from build123d import *

# Parameters (mm, degrees)
SKETCH1_W           = 4.75
SKETCH1_H           = 10
SKETCH1_W_2         = 195.25
SKETCH1_H_2         = 75
SKETCH1_W_3         = 10
SKETCH1_H_3         = 6
SKETCH1_H_4         = 35
BOSS_EXTRUDE1_DEPTH = 4.75
SKETCH3_W           = 4.75
SKETCH3_H           = 35
CUT_EXTRUDE2_DEPTH  = 4.75
SKETCH4_W           = 3
SKETCH4_H           = 16
SKETCH4_W_2         = 5.5
SKETCH4_H_2         = 3
CUT_EXTRUDE3_DEPTH  = 4.75
SKETCH5_W           = 10
SKETCH5_H           = 4.75
CUT_EXTRUDE4_DEPTH  = 214.652901923
SKETCH6_R           = 1.5
CUT_EXTRUDE5_DEPTH  = 214.652901923
SKETCH7_W           = 10
SKETCH7_H           = 4.75
BOSS_EXTRUDE2_DEPTH = 4.75
SKETCH8_R           = 2.5
CUT_EXTRUDE6_DEPTH  = 216.366257803
SKETCH9_W           = 3
SKETCH9_H           = 16
SKETCH9_W_2         = 5.5
SKETCH9_H_2         = 3
CUT_EXTRUDE7_DEPTH  = 10


with BuildPart() as part:
    # Sketch1 → Boss-Extrude1 (new body)
    with BuildSketch(Plane(origin=(0, 0, 0), x_dir=(1, 0, 0), z_dir=(0, 1, 0))):
        with Locations((-197.625, 60)):
            Rectangle(SKETCH1_W, SKETCH1_H)
        with Locations((-97.625, 37.5)):
            Rectangle(SKETCH1_W_2, SKETCH1_H_2)
        with Locations((-140.25, -3)):
            Rectangle(SKETCH1_W_3, SKETCH1_H_3)
        with Locations((-97.625, -3)):
            Rectangle(SKETCH1_W_3, SKETCH1_H_3)
        with Locations((-55, -3)):
            Rectangle(SKETCH1_W_3, SKETCH1_H_3)
        with Locations((2.375, 17.5)):
            Rectangle(SKETCH1_W, SKETCH1_H_4)
        with Locations((2.375, 50)):
            Rectangle(SKETCH1_W, SKETCH1_H)
        with Locations((2.375, 70)):
            Rectangle(SKETCH1_W, SKETCH1_H)
        with Locations((-197.625, 40)):
            Rectangle(SKETCH1_W, SKETCH1_H)
    extrude(amount=BOSS_EXTRUDE1_DEPTH)

    # Sketch3 → Cut-Extrude2 (cut)
    with BuildSketch(Plane(origin=(0, 4.75, 0), x_dir=(1, 0, 0), z_dir=(0, 1, 0))):
        with BuildLine():
            Line((-180.25, 35), (-195.25, 35))
            Line((-195.25, 35), (-195.25, 0))
            Line((-195.25, 0), (-150.25, 0))
            Line((-150.25, 0), (-150.25, 5))
            ThreePointArc((-150.25, 5), (-159.036796564, 26.213203436), (-180.25, 35))
        make_face()
        with BuildLine():
            Line((-45, 0), (0, 0))
            Line((0, 0), (0, 35))
            Line((0, 35), (-15, 35))
            ThreePointArc((-15, 35), (-36.213203436, 26.213203436), (-45, 5))
            Line((-45, 5), (-45, 0))
        make_face()
        with Locations((2.375, 17.5)):
            Rectangle(SKETCH3_W, SKETCH3_H)
    extrude(amount=-CUT_EXTRUDE2_DEPTH, mode=Mode.SUBTRACT)

    # Sketch4 → Cut-Extrude3 (cut)
    with BuildSketch(Plane(origin=(0, 4.75, 0), x_dir=(1, 0, 0), z_dir=(0, 1, 0))):
        with Locations((-118.9375, 8)):
            Rectangle(SKETCH4_W, SKETCH4_H)
        with Locations((-76.3125, 8)):
            Rectangle(SKETCH4_W, SKETCH4_H)
        with Locations((-118.9375, 7.5)):
            Rectangle(SKETCH4_W_2, SKETCH4_H_2)
        with Locations((-76.3125, 7.5)):
            Rectangle(SKETCH4_W_2, SKETCH4_H_2)
    extrude(amount=-CUT_EXTRUDE3_DEPTH, mode=Mode.SUBTRACT)

    # Sketch5 → Cut-Extrude4 (cut, through all)
    with BuildSketch(Plane.XZ):
        with Locations((-155.25, -37.375)):
            Rectangle(SKETCH5_W, SKETCH5_H)
        with Locations((-97.625, -37.375)):
            Rectangle(SKETCH5_W, SKETCH5_H)
        with Locations((-40, -37.375)):
            Rectangle(SKETCH5_W, SKETCH5_H)
    extrude(amount=-CUT_EXTRUDE4_DEPTH, mode=Mode.SUBTRACT)

    # Sketch6 → Cut-Extrude5 (cut, through all)
    with BuildSketch(Plane.XZ):
        with Locations(Location((-68.8125, -37.375, 0), (0, 0, 270))):
            Circle(SKETCH6_R)
        with Locations(Location((-126.4375, -37.375, 0), (0, 0, 270))):
            Circle(SKETCH6_R)
    extrude(amount=-CUT_EXTRUDE5_DEPTH, mode=Mode.SUBTRACT)

    # Sketch7 → Boss-Extrude2 (add)
    with BuildSketch(Plane(origin=(0, 4.75, 0), x_dir=(1, 0, 0), z_dir=(0, 1, 0))):
        with Locations((-175.25, 77.375)):
            Rectangle(SKETCH7_W, SKETCH7_H)
        with Locations((-123.5, 77.375)):
            Rectangle(SKETCH7_W, SKETCH7_H)
        with Locations((-71.75, 77.375)):
            Rectangle(SKETCH7_W, SKETCH7_H)
        with Locations((-20, 77.375)):
            Rectangle(SKETCH7_W, SKETCH7_H)
    extrude(amount=-BOSS_EXTRUDE2_DEPTH)

    # Sketch8 → Cut-Extrude6 (cut, through all)
    with BuildSketch(Plane.XZ):
        with Locations(Location((-97.625, -60, 0), (0, 0, 270))):
            Circle(SKETCH8_R)
    extrude(amount=-CUT_EXTRUDE6_DEPTH, mode=Mode.SUBTRACT)

    # Sketch9 → Cut-Extrude7 (cut)
    with BuildSketch(Plane.XZ):
        with Locations((-97.625, -67)):
            Rectangle(SKETCH9_W, SKETCH9_H)
        with Locations((-97.625, -67.5)):
            Rectangle(SKETCH9_W_2, SKETCH9_H_2)
    extrude(amount=-CUT_EXTRUDE7_DEPTH, mode=Mode.SUBTRACT)


solid = part.part
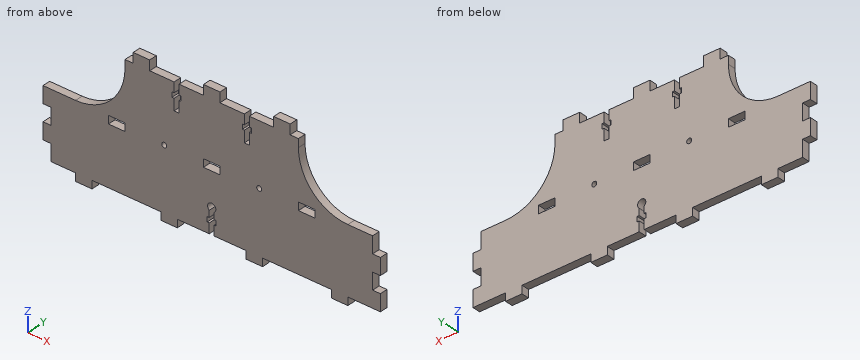
Build history of the part. All positions in model axes, mm. Give positions to 0.01 mm unless a question says otherwise; leave off trailing zeros. Write each loop counter-clockwise with the first axis right and the second up, starting at its lowest first coordinate (ties: lowest second). Pieces come first, ordered by that corner, then holes. Notation, with made-up numbers: (36.25, -14.75) - (76.25, -14.75) arc R31 ccw to (76.25, 19.25) - close; hole circle Ø3 at (-36.5, 56.5). An arc over 180 degrees is marked (long way). Use one line per item in the form item = value. Start each with the question number.
1. Probe line 1 (X direction, y = 2.05, z = -60) (3 decimals); line 2 (X direction, y = 1.85, z = -72) (3 decimals); line 3 (X direction, y = 0.65, z = -35.5) (3 decimals). List the from-to ranges inside material, lowest first. Write a range as [from, to].
2. Band-saw the part on A-A on z = -60. Write the cut outline in (x, y) (3 decimals).
3. Band-saw the part on C-C on x = -131. Write the cut outline in (y, z).
4. Band-saw the part on B-B on z = -48. Write the cut outline in (x, y).
5. Drop flat-ended pins along their axis: pin 1 Ø1 at (x, y) = (-113, 3) entering from -Z; pin 2 Ø1.4 at (x, y) = (-148, 3) entering from +Z; pin 3 Ø1.5 at (x, y) = (-26, 4) entering from +Z. Give the stop position or say it passes through.
6. Band-saw the part on D-D on y = 0.85. Count the separate pieces of the cut face and the enclosed holes in it, plus the area to 3 significant figures.
Conclusion:
q1.line_1 = [-200, -100.125], [-95.125, 0]
q1.line_2 = [-195.25, -99.125], [-96.125, 4.75]
q1.line_3 = [-200, -160.25], [-150.25, -102.625], [-92.625, -45], [-35, 0]
q2.outline = (-200, 0) - (-100.125, 0) - (-100.125, 4.75) - (-200, 4.75) - close; (-95.125, 0) - (0, 0) - (0, 4.75) - (-95.125, 4.75) - close
q3.outline = (0, -75) - (4.75, -75) - (4.75, 0) - (0, 0) - close
q4.outline = (-195.25, 0) - (4.75, 0) - (4.75, 4.75) - (-195.25, 4.75) - close
q5.pin_1 = -75
q5.pin_2 = 0
q5.pin_3 = -32.6
q6.separate_pieces = 1
q6.enclosed_holes = 5
q6.area = 12,100 mm²
